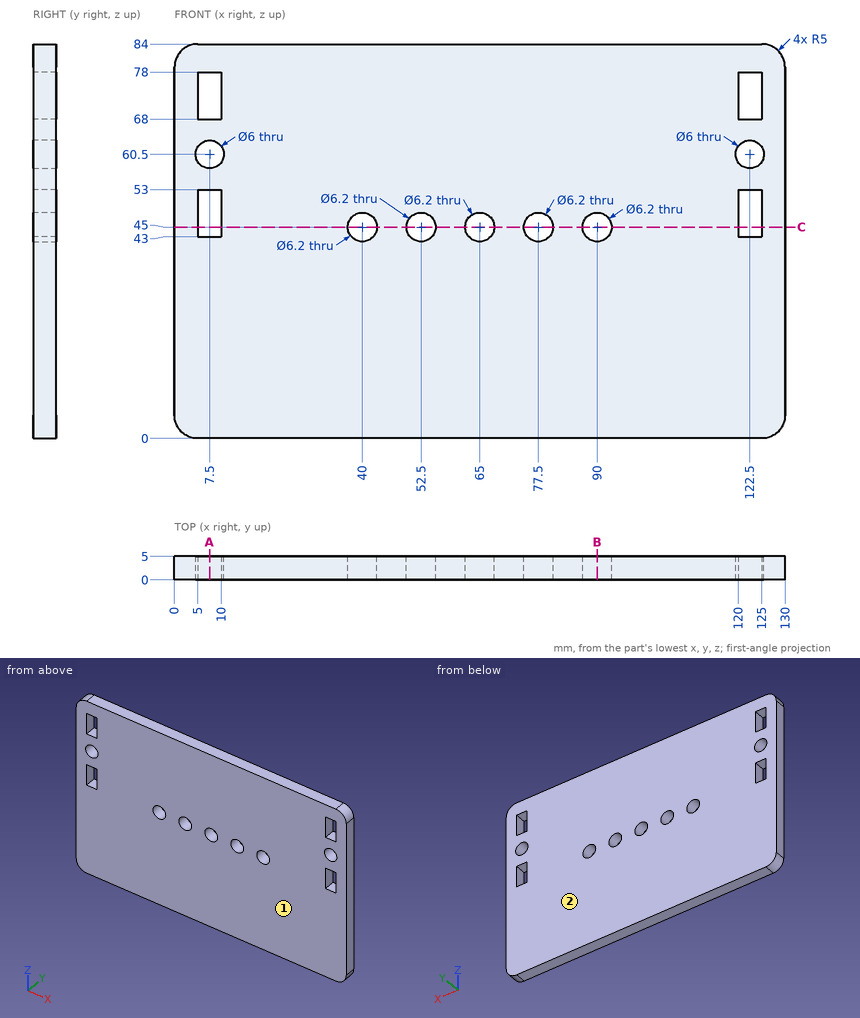
Design review of the part shown in the three views and the two pictorial views. Dimensions are in mm from the part's minimum x, y and z. Round coordinates to 2 decimals unless told otherwise and drop trailing zeros. Order: outer loops, then holes, each group sorted by start corner. A loop starts at its lowest first (then second) coordinate and runs counter-clockwise, first axis right, second up. Notation, with made-up numbers: (76, 70.5) - (124, 70.5) arc R17 ccw to (124, 96.5) - close; hole circle Ø2 at (89.5, -7). An arc over 180 degrees is marked (long way). Answer in a Markdown table with one row per item.
(1) Mouldability with a two-part tool opening along Y and no side actions: class the marked faces 1 and 2 as released by +Y, released by -Y, zero draft, split by the parting line, or undercut.
Result set:
| item | result |
|---|---|
| face 1 | released by -Y |
| face 2 | released by +Y |
(2) Take a section at A-A on x = 7.5. Write out the cut boundary in (y, z), plus the area to 3 significant figures.
Result set:
| item | result |
|---|---|
| outline | (0, 0) - (5, 0) - (5, 43) - (0, 43) - close; (0, 53) - (5, 53) - (5, 57.5) - (0, 57.5) - close; (0, 63.5) - (5, 63.5) - (5, 68) - (0, 68) - close; (0, 78) - (5, 78) - (5, 84) - (0, 84) - close |
| area | 290 mm2 |
(3) Take a section at B-B on x = 90. Write out the cut boundary in (y, z).
Result set:
| item | result |
|---|---|
| outline | (0, 0) - (5, 0) - (5, 41.9) - (0, 41.9) - close; (0, 48.1) - (5, 48.1) - (5, 84) - (0, 84) - close |
(4) For line 1 (X direction, y = 2.4, z = 49.5); line 2 (X direction, y = 3.45, z = 60.5); line 3 (Z direction, x = 89, y = 0.45), list the stretches that pass through material, from the lowest coordinate up. Write a range as from..to.
Result set:
| item | result |
|---|---|
| line 1 | x = 0..5, 10..120, 125..130 |
| line 2 | x = 0..4.5, 10.5..119.5, 125.5..130 |
| line 3 | z = 0..42.07, 47.93..84 |
(5) Take a section at C-C on z = 45. Count the separate pieces of the cut face and the enclosed holes in it, plus the area to 3 significant figures.
Result set:
| item | result |
|---|---|
| separate pieces | 8 |
| enclosed holes | 0 |
| area | 445 mm2 |
